Geometry: see drawing. Coordinates: mm, zero at the bounding-box minimum. Give positions to 0.01 mm unless a question says otherwise; leave off trailing zeros. Loops run counter-clockwise (first coordinate to the right, second up) from the corner with the lowest first, then second, coordinate; pieces in that order, holes last. Notation, with made-up numbers: M 74,57.5 L 109,57.5 A10 cw 109,75.5 Z; hole C -22.75,-11 d5. An arc over 180 degrees is marked long. Answer in a Markdown table with one row per item.
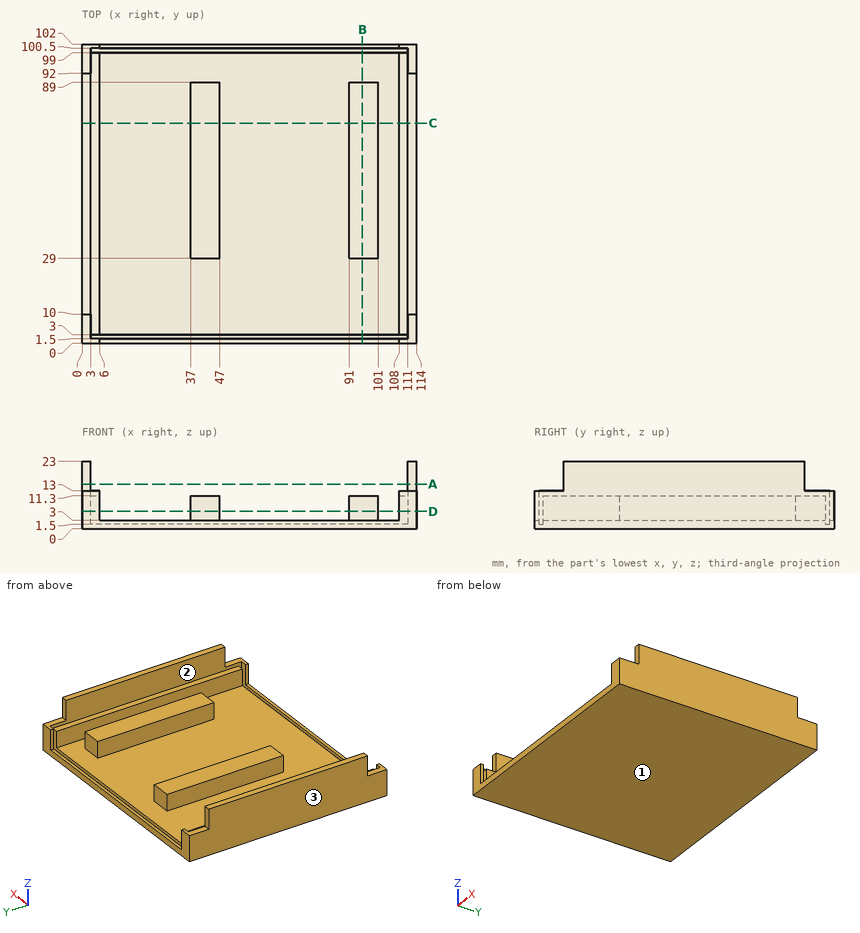
1) Section A-A, the plane z = 15.25. Return loops of the section in (x, y).
Reply:
| item | result |
|---|---|
| outline | M 0,10 L 3,10 L 3,92 L 0,92 Z; M 111,10 L 114,10 L 114,92 L 111,92 Z |
2) Material intervals for L1, parallel to X at y = 79, z = 6; L2, parallel to X at y = 25.5, z = 14; L3, parallel to X at y = 14, z = 7.5, sorted ascending.
Reply:
| item | result |
|---|---|
| L1 | x = 0 to 6, 37 to 47, 91 to 101, 108 to 114 |
| L2 | x = 0 to 3, 111 to 114 |
| L3 | x = 0 to 6, 108 to 114 |
3) Section D-D, the plane z = 6. Count the separate pieces of the cut face and the enclosed holes in it, then the cut area to 3 significant figures.
Reply:
| item | result |
|---|---|
| separate pieces | 4 |
| enclosed holes | 0 |
| area | 2,410 mm² |
4) Pull-direction query (X, two-part tool) for the marked faces 1, 2 and 3; classes: released by +X, released by -X, zero draft, split by the parting line, or undercut.
Reply:
| item | result |
|---|---|
| face 1 | zero draft |
| face 2 | undercut |
| face 3 | released by -X |
5) Section B-B, the plane x = 95.5. Return loops of the section in (y, z).
Reply:
| item | result |
|---|---|
| outline | M 0,0 L 102,0 L 102,3 L 100.5,3 L 100.5,1.5 L 99,1.5 L 99,3 L 89,3 L 89,11.3 L 29,11.3 L 29,3 L 3,3 L 3,1.5 L 1.5,1.5 L 1.5,3 L 0,3 Z |
6) Pin query (flat end, axial travel): pin 1 Ø6.5 at (x, y) = (111.5, 95.5) entering from +Z; pin 2 Ø5 at (x, z) = (43.5, 8.5) entering from +Y; pin 3 Ø0.8 at (x, y) = (58, 2.5) entering from +Z. Return the tip coordinate at first contact, or that it passes through.
Reply:
| item | result |
|---|---|
| pin 1 | stops at z = 13 |
| pin 2 | stops at y = 89 |
| pin 3 | stops at z = 1.5 |
7) Section C-C, the plane y = 75. Return loops of the section in (x, z).
Reply:
| item | result |
|---|---|
| outline | M 0,0 L 114,0 L 114,23 L 111,23 L 111,11.3 L 108,11.3 L 108,3 L 101,3 L 101,11.3 L 91,11.3 L 91,3 L 47,3 L 47,11.3 L 37,11.3 L 37,3 L 6,3 L 6,11.3 L 3,11.3 L 3,23 L 0,23 Z |
